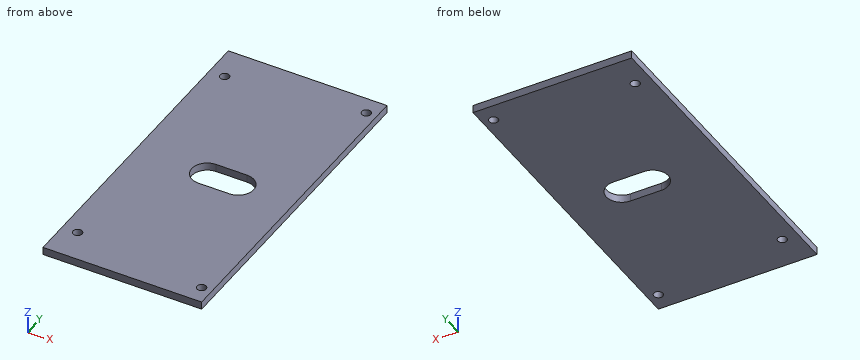
```python
from build123d import *

# Parameters (mm, degrees)
SKETCH1_W           = 61.5
SKETCH1_H           = 126
SKETCH1_R           = 1.75
BOSS_EXTRUDE1_DEPTH = 3
CUT_EXTRUDE1_REACH  = 90.092


with BuildPart() as part:
    # Sketch1 → Boss-Extrude1 (new body)
    with BuildSketch(Plane.XY):
        with Locations((-30.75, 0)):
            Rectangle(SKETCH1_W, SKETCH1_H)
        with Locations((-4, 56)):
            Circle(SKETCH1_R, mode=Mode.SUBTRACT)
        with Locations((-55.5, 50)):
            Circle(SKETCH1_R, mode=Mode.SUBTRACT)
        with Locations(Location((-4, -56, 0), (0, 0, 180))):
            Circle(SKETCH1_R, mode=Mode.SUBTRACT)
        with Locations(Location((-55.5, -50, 0), (0, 0, 180))):
            Circle(SKETCH1_R, mode=Mode.SUBTRACT)
    extrude(amount=BOSS_EXTRUDE1_DEPTH)

    # Sketch2 → Cut-Extrude1 (cut, up to next)
    with BuildSketch(Plane.XY.offset(3), mode=Mode.PRIVATE) as cut_extrude1_sk1:
        with BuildLine():
            Line((-33.75, 6), (-21.75, 6))
            ThreePointArc((-21.75, 6), (-15.75, 0), (-21.75, -6))
            Line((-21.75, -6), (-33.75, -6))
            ThreePointArc((-33.75, -6), (-39.75, 0), (-33.75, 6))
        make_face()
    cut_extrude1_tool1 = extrude(cut_extrude1_sk1.sketch, amount=-CUT_EXTRUDE1_REACH, mode=Mode.PRIVATE) & part.part
    add(cut_extrude1_tool1.solids().sort_by_distance((-27.75, 0, 3))[0], mode=Mode.SUBTRACT)


solid = part.part
```
Input: part model. Units: mm. Frame: model coordinates. Coordinates: 2 decimals unless noted, no trailing zeros. Loops run counter-clockwise (first coordinate to the right, second up) from the corner with the lowest first, then second, coordinate; pieces in that order, holes last. Notation, with made-up numbers: M 50.25,83 L 62.25,83 A19 cw 62.25,92 Z; hole C 71,-1 d1. An arc over 180 degrees is marked long. Answer in a Markdown table with one row per item.
1. Section C-C, the plane z = 1.1. Output: boundary loops of the cut face in (x, y).
Response:
| item | result |
|---|---|
| outline | M -61.5,-63 L 0,-63 L 0,63 L -61.5,63 Z; hole C -55.5,-50 d3.5; hole C -55.5,50 d3.5; hole M -33.75,-6 L -21.75,-6 A6 ccw -21.75,6 L -33.75,6 A6 ccw Z; hole C -4,-56 d3.5; hole C -4,56 d3.5 |
2. Section D-D, the plane x = -3.5. Output: boundary loops of the cut face in (y, z), then the cut area to 3 significant figures.
Response:
| item | result |
|---|---|
| outline | M -63,0 L -57.68,0 L -57.68,3 L -63,3 Z; M -54.32,0 L 54.32,0 L 54.32,3 L -54.32,3 Z; M 57.68,0 L 63,0 L 63,3 L 57.68,3 Z |
| area | 358 mm2 |
3. Section B-B, the plane y = -50. Output: boundary loops of the cut face in (x, z).
Response:
| item | result |
|---|---|
| outline | M -61.5,0 L -57.25,0 L -57.25,3 L -61.5,3 Z; M -53.75,0 L 0,0 L 0,3 L -53.75,3 Z |
4. Material intervals for line 1 (Y direction, x = -55.5, z = 1.1); line 2 (Y direction, x = -4, z = 2.15); line 3 (Y direction, x = -30, z = 1.2), sorted ascending.
Response:
| item | result |
|---|---|
| line 1 | y = -63 to -51.75, -48.25 to 48.25, 51.75 to 63 |
| line 2 | y = -63 to -57.75, -54.25 to 54.25, 57.75 to 63 |
| line 3 | y = -63 to -6, 6 to 63 |
5. Section A-A, the plane x = -32. Output: boundary loops of the cut face in (y, z).
Response:
| item | result |
|---|---|
| outline | M -63,0 L -6,0 L -6,3 L -63,3 Z; M 6,0 L 63,0 L 63,3 L 6,3 Z |
